Autodesk Inventor part; units mm, degrees
ref_plane "YZ Plane" through (0, 0, 0) normal (1, 0, 0) x (0, 1, 0)
ref_plane "XZ Plane" through (0, 0, 0) normal (0, 1, 0) x (-1, 0, 0)
ref_plane "XY Plane" through (0, 0, 0) normal (0, 0, 1) x (1, 0, 0)
sketch "Sketch1" plane through (0, 0, 0) normal (0, 1, 0) x (-1, 0, 0)
  line L0 (0, 0) -> (0, -42)
  line L1 (0, -42) -> (12, -42)
  line L2 (12, -42) -> (12, 0)
  line L3 (12, 0) -> (0, 0)
  line L4 (0, -21) -> (0, -26)
  line L5 (0, -21) -> (0, -16)
  line L6 (0, -16) -> (0, -19)
  line L7 (0, -16) -> (0, -13)
  line L8 (0, -26) -> (0, -23)
  line L9 (0, -26) -> (0, -29)
  line L10 (0, -29) -> (12, -29)
  line L11 (0, -13) -> (12, -13)
  line L12 (6.4, -16) -> (12, -16)
  line L13 (6.4, -26) -> (12, -26)
  line L14 (12, -16) -> (8, -16)
  circle A0 centre (8, -16) radius 1.6
  circle A1 centre (8, -26) radius 1.6
  line L15 (12, -26) -> (8, -26)
  dimension "d9" = 3.2
  dimension "d10" = 3.2
  dimension "d0" = 42
  dimension "d1" = 12
  dimension "d2" = 5
  dimension "d3" = 5
  dimension "d4" = 3
  dimension "d5" = 3
  dimension "d6" = 3
  dimension "d7" = 3
  dimension "d8" = 4
extrude "Extrusion1" add sketch "Sketch1" along normal blind 15
sketch "Sketch2" plane through (0, 0, 0) normal (0, -1, 0) x (1, 0, 0)
  line L0 (-12, 0) -> (-12, -42)
  line L1 (-12, -42) -> (-12, 0)
  line L2 (-12, -21) -> (-42, -21)
  circle A0 centre (-42, -21) radius 3.5
  arc A1 (-47, -35.1421) -> (-47, -6.8579) centre (-42, -21) ccw
  line L3 (-42, -21) -> (-47, -21)
  line L4 (-47, -21) -> (-47, -35.1421)
  line L5 (-47, -21) -> (-47, -6.8579)
  line L6 (-42, -36) -> (-12, -42)
  line L7 (-42, -6) -> (-12, 0)
  line L8 (-12, -42) -> (0, -42)
  line L9 (0, -42) -> (0, 0)
  line L10 (0, 0) -> (0, -42)
  line L11 (0, 0) -> (-12, 0)
  circle A2 centre (-8, -16) radius 1.6
  circle A3 centre (-8, -16) radius 1.6
  circle A4 centre (-8, -26) radius 1.6
  circle A5 centre (-8, -26) radius 1.6
  line L12 (-12, -42) -> (-12, -36.5)
  line L13 (-12, 0) -> (-12, -5.5)
  line L14 (-17, -6.5) -> (-32.2985, -9.5597)
  line L15 (-32.2985, -32.4403) -> (-17, -35.5)
  circle A6 centre (-42, -21) radius 5
  line L16 (-12, -21) -> (-17, -21)
  line L17 (-17, -16) -> (-17, -6.5)
  line L18 (-17, -26) -> (-17, -35.5)
  line L19 (-42, -16) -> (-33.9223, -16)
  line L20 (-27.8579, -16) -> (-12, -16)
  line L21 (-42, -26) -> (-33.9223, -26)
  line L22 (-27.8579, -26) -> (-12, -26)
  arc A7 (-47, -29.3703) -> (-47, -12.6297) centre (-42, -21) ccw
  point P0 (-47, -12.9223)
  point P1 (-47, -29.0777)
  dimension "d13" = 30
  dimension "d14" = 7
  dimension "d16" = 30
  dimension "d17" = 5
  dimension "d30" = 5.5
  dimension "d31" = 5.5
  dimension "d32" = 10
  dimension "d33" = 5
  dimension "d36" = 19.5
extrude "Extrusion2" add sketch "Sketch2" along normal blind 10 contours L11 L9 L8 L0 | L0 L20 L17 L14 A1 L7 | A1 L2 A7 L5 | L0 L2 A1 L20 | L14 L17 L20 A1 | L0 L22 A1 L2 | A7 L2 A6 L5 | L6 A1 L15 L18 L22 L0 | A1 L4 A7 L2 | A6 L2 A0 L3 | A6 L2 A7 L4 | L3 A0 L2 A6 | L18 L15 A1 L22
sketch "Sketch3" plane through (0, 15, 0) normal (1, 0, 0) x (0, 0, -1)
  line L0 (0, -15) -> (42, -15)
  line L1 (42, -15) -> (0, -15)
  line L2 (21, -15) -> (34, -15)
  line L3 (34, -15) -> (34, -8)
  line L4 (21, -15) -> (8, -15)
  line L5 (8, -15) -> (8, -8)
  circle A0 centre (8, -8) radius 2.65
  circle A1 centre (34, -8) radius 2.65
  dimension "d22" = 13
  dimension "d23" = 7
  dimension "d24" = 13
  dimension "d25" = 7
  dimension "d26" = 5.3
  dimension "d27" = 5.3
extrude "Extrusion4" cut sketch "Sketch3" against normal blind 15
extrude "Extrusion5" cut sketch "Sketch2" along normal blind 15 contours L14 L17 L20 A1 | L18 L15 A1 L22
extrude "Extrusion6" cut sketch "Sketch2" along normal blind 6 contours A7 L2 A6 L5 | A6 L2 A0 L3 | A6 L2 A7 L4 | L3 A0 L2 A6
properties part number "servo_clip_holder2"
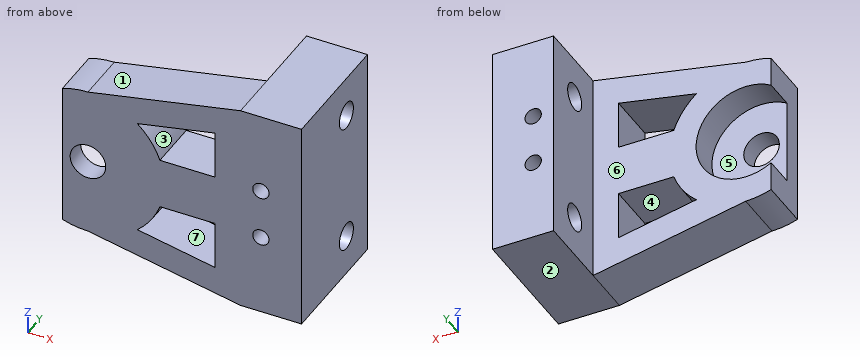
CAD build for the part. Positions are in the model's coordinates, mm. Face numbers are marked on the shaded views. A direction names the side the tool comes from. Coordinates: 2 decimals unless noted, no trailing zeros. Order: outer loops, then holes, each group sorted by start corner. A loop starts at its lowest first (then second) coordinate and runs counter-clockwise, first axis right, second up. Notation, with made-up numbers: (31.25, 22.25) -> (66.25, 22.25) arc R17 cw to (66.25, 55.25) -> close; hole circle Ø8 at (18.5, 7). An arc over 180 degrees is marked (long way). Answer in a Markdown table with one row per item.
1) Mould opens along X. For the marked faces 1, 2, 3 and 4 say: pulls with the +X half, pulls with the -X half, needs draft (parallel to the pull), parting line crosses it, or undercut.
Check values:
| item | result |
|---|---|
| face 1 | pulls with the -X half |
| face 2 | needs draft |
| face 3 | undercut |
| face 4 | undercut |
2) Which spindle directions (+Z, -Z, +X, -X, +Y, -Y) get a long thin tool onto all of the face, cutting with end or side? Do the marked faces 5, 6 and 7. Say none if no direction does.
Check values:
| item | result |
|---|---|
| face 5 | +Y |
| face 6 | +Z, -Z, -X, +Y |
| face 7 | +Y, -Y |
3) Band-saw the part on B-B (y = 7). List the corners of the cut face in (x, z).
Check values:
| item | result |
|---|---|
| outline | (-12, -42) -> (0, -42) -> (0, -36.65) -> (-12, -36.65) -> close; (-12, -31.35) -> (0, -31.35) -> (0, -10.65) -> (-12, -10.65) -> close; (-12, -5.35) -> (0, -5.35) -> (0, 0) -> (-12, 0) -> close; hole circle Ø3.2 at (-8, -26); hole circle Ø3.2 at (-8, -16) |
4) Band-saw the part on A-A (x = -8). List the corners of the cut face in (y, z), and give its area (3 significant figures).
Check values:
| item | result |
|---|---|
| outline | (-10, -42) -> (15, -42) -> (15, -27.6) -> (-10, -27.6) -> close; (-10, -24.4) -> (15, -24.4) -> (15, -17.6) -> (-10, -17.6) -> close; (-10, -14.4) -> (15, -14.4) -> (15, 0) -> (-10, 0) -> close; hole circle Ø5.3 at (7, -34); hole circle Ø5.3 at (7, -8) |
| area | 846 mm2 |
5) Band-saw the part on D-D (y = 3). List the corners of the cut face in (x, z), and give its area (3 significant figures).
Check values:
| item | result |
|---|---|
| outline | (-12, -42) -> (0, -42) -> (0, 0) -> (-12, 0) -> close; hole circle Ø3.2 at (-8, -26); hole circle Ø3.2 at (-8, -16) |
| area | 488 mm2 |
6) Flat gauge pins, fed straight in: P1, Ø11, axis at x = -25, y = -6, coming from the -Z side; P2, Ø1.5, axis at y = 4, z = -27.5, coming from the -X side; P3, Ø6, axis at x = -29.5, y = 1, coming from the -Z side. Where does each tip first touch, or does it go through?
Check values:
| item | result |
|---|---|
| P1 | z = -40.5 |
| P2 | x = -12 |
| P3 | z = -39.07 |
7) Drill centre lines: line 1 (Z direction, x = -4, y = 7); line 2 (X direction, y = 3.25, z = -26); line 3 (Z direction, x = -42, y = -7.05). Where is each one in solid material? Low to high.
Check values:
| item | result |
|---|---|
| line 1 | -42 to -36.65, -31.35 to -10.65, -5.35 to 0 |
| line 2 | -12 to -9.6, -6.4 to 0 |
| line 3 | -36 to -24.5, -17.5 to -6 |
8) Band-saw the part on C-C (z = -8). List the corners of the cut face in (x, y), and give its area (3 significant figures).
Check values:
| item | result |
|---|---|
| outline | (-47, -10) -> (-24.5, -10) -> (-24.5, 0) -> (-47, 0) -> close; (-17, -10) -> (0, -10) -> (0, 4.35) -> (-12, 4.35) -> (-12, 0) -> (-17, 0) -> close; (-12, 9.65) -> (0, 9.65) -> (0, 15) -> (-12, 15) -> close |
| area | 511 mm2 |
